Verification items for the finished model (mm, model axes). A direction names the side the tool comes from. Coordinates: 2 decimals unless noted, no trailing zeros. Order: outer loops, then holes, each group sorted by start corner. A loop starts at its lowest first (then second) coordinate and runs counter-clockwise, first axis right, second up. Notation, with made-up numbers: M 0.5,-25 L 21.5,-25 A7 cw 21.5,-13 Z; hole C 70.5,12 d10. An arc over 180 degrees is marked long. Return JSON: item names as keys, results as strings. Group by question number.
1. Section check B-B, the plane x = -1.5. Give the number of separate pieces and of enclosed holes in the cut face, plus the area to 3 significant figures.
2. Mould release check, pull along Y, two halves, no side actions. Record for faces 4 (the flat face through (-1, 1.1, -1)), 5 (the flat face through (1, -4.1, -1)), 6 (the flat face through (0, -1, -3.3)), 7 (the cylindrical face through (-1.66, -2.62, 1.17)): +Y half, -Y half, draft (parallel to the pull), parting line (faces both ways), or undercut.
3. Section check A-A, the plane z = 0.8. Record the cut outline in (x, y), plus the area to 3 significant figures.
4. Section check C-C, the plane y = -1.25. Record the cut outline in (x, z).
5. Section check D-D, the plane z = 3.5. Record the cut outline in (x, y), plus the area to 3 significant figures.
6. Material ranges on line 1 along Y through (x, z) = (-1, -3.5); line 2 along X through (y, z) = (1.95, 0.8); line 3 along Y through (x, z) = (-1.75, 0.5), recorded low to high.
7. Set-up check for faces 1 (the flat face through (0, 2, 3.9)), 2 (the flat face through (0, -3, -3.3)), 3 (the flat face through (0, 0, -2.3)): record each of +Z, -Z, +X, -X, +Y, -Y from which the full face is reachable in a straight line by a thin tool's end or side.
8. Gauge pin test, flat ends, axial feed: pin 1 (1 mm diameter, centred on x = 1.5, y = 1, fed in from -Z); pin 2 (0.6 mm diameter, centred on x = 1.5, y = 2.5, fed in from -Z); pin 3 (1 mm diameter, centred on x = 1, y = 0, fed in from +Z); pin 4 (1.5 mm diameter, centred on x = 0.5, z = 1, fed in from -Y). Record the tip position at first contact, or that the pin passes through.
```python
from build123d import *

# Parameters (mm, degrees)
SKETCH1_W           = 8.3
SKETCH1_H           = 7.8
BOSS_EXTRUDE1_DEPTH = 4.1
CUT_EXTRUDE1_DEPTH  = 11.045396956
SKETCH4_W           = 6.2
SKETCH4_H           = 2.2
CUT_EXTRUDE2_DEPTH  = 6.2
SKETCH5_R           = 1.7
CUT_EXTRUDE3_DEPTH  = 10.983611571
FILLET1_R           = 0.5


with BuildPart() as part:
    # Sketch1 → Boss-Extrude1 (new, symmetric)
    with BuildSketch(Plane(origin=(0, 0, 0), x_dir=(1, 0, 0), z_dir=(0, 1, 0))):
        Rectangle(SKETCH1_W, SKETCH1_H)
    extrude(amount=BOSS_EXTRUDE1_DEPTH, both=True)

    # Sketch2 → Cut-Extrude1 (cut, through all)
    with BuildSketch(Plane.ZY.offset(4.15)):
        Polygon((-8.9, 3.6), (-3.3, 3.6), (-3.3, 2.4), (-3.9, 2.4), (-3.9, 1.6), (-3.3, 1.6), (-3.3, 0.4), (-3.9, 0.4), (-3.9, -0.4), (-3.3, -0.4), (-3.3, -1.6), (-3.9, -1.6), (-3.9, -2.4), (-3.3, -2.4), (-3.3, -3.6), (-8.9, -3.6), align=None)
    extrude(amount=-CUT_EXTRUDE1_DEPTH, mode=Mode.SUBTRACT)

    # Sketch4 → Cut-Extrude2 (cut)
    with BuildSketch(Plane.XY.offset(3.9)):
        Rectangle(SKETCH4_W, SKETCH4_H)
    extrude(amount=-CUT_EXTRUDE2_DEPTH, mode=Mode.SUBTRACT)

    # Sketch5 → Cut-Extrude3 (cut, through all)
    with BuildSketch(Plane.XZ.offset(4.1)):
        with Locations(Location((0, 0.8, 0), (0, 0, 270))):
            Circle(SKETCH5_R)
    extrude(amount=-CUT_EXTRUDE3_DEPTH, mode=Mode.SUBTRACT)

    # Fillet1
    fillet1_edges = [part.edges().sort_by_distance(p)[0] for p in [
        (4.15, 4.1, 0),
        (4.15, -4.1, 0),
        (-4.15, 4.1, 0),
        (-4.15, -4.1, 0),
    ]]
    fillet(fillet1_edges, radius=FILLET1_R - 0.0001)  # a hair under: the kernel refuses the full size


solid = part.part
```
Answers follow:
{
 "1": {"separate pieces": "3", "enclosed holes": "0", "area": "37.8 mm^2"},
 "2": {"face 4": "undercut", "face 5": "-Y half", "face 6": "undercut", "face 7": "draft"},
 "3": {"outline": "M -4.15,-3.6 A0.5 ccw -3.65,-4.1 L -1.7,-4.1 L -1.7,-1.1 L -3.1,-1.1 L -3.1,1.1 L -1.7,1.1 L -1.7,4.1 L -3.65,4.1 A0.5 ccw -4.15,3.6 Z; M 1.7,-4.1 L 3.65,-4.1 A0.5 ccw 4.15,-3.6 L 4.15,3.6 A0.5 ccw 3.65,4.1 L 1.7,4.1 L 1.7,1.1 L 3.1,1.1 L 3.1,-1.1 L 1.7,-1.1 Z", "area": "33.8 mm^2"},
 "4": {"outline": "M -4.15,-3.3 L 4.15,-3.3 L 4.15,3.9 L -4.15,3.9 Z; hole C 0,0.8 d3.4"},
 "5": {"outline": "M -4.15,-3.6 A0.5 ccw -3.65,-4.1 L 3.65,-4.1 A0.5 ccw 4.15,-3.6 L 4.15,3.6 A0.5 ccw 3.65,4.1 L -3.65,4.1 A0.5 ccw -4.15,3.6 Z; hole M -3.1,-1.1 L 3.1,-1.1 L 3.1,1.1 L -3.1,1.1 Z", "area": "54.2 mm^2"},
 "6": {"line 1": "-4.1 to -3.6, -2.4 to -1.6, -0.4 to 0.4, 1.6 to 2.4, 3.6 to 4.1", "line 2": "-4.15 to -1.7, 1.7 to 4.15", "line 3": "-4.1 to -1.1, 1.1 to 4.1"},
 "7": {"face 1": "+Z, +X, -X, +Y, -Y", "face 2": "-Z, +X, -X", "face 3": "+Z"},
 "8": {"pin 1": "z = -3.3", "pin 2": "z = -3.9", "pin 3": "z = -2.3", "pin 4": "through"}
}
